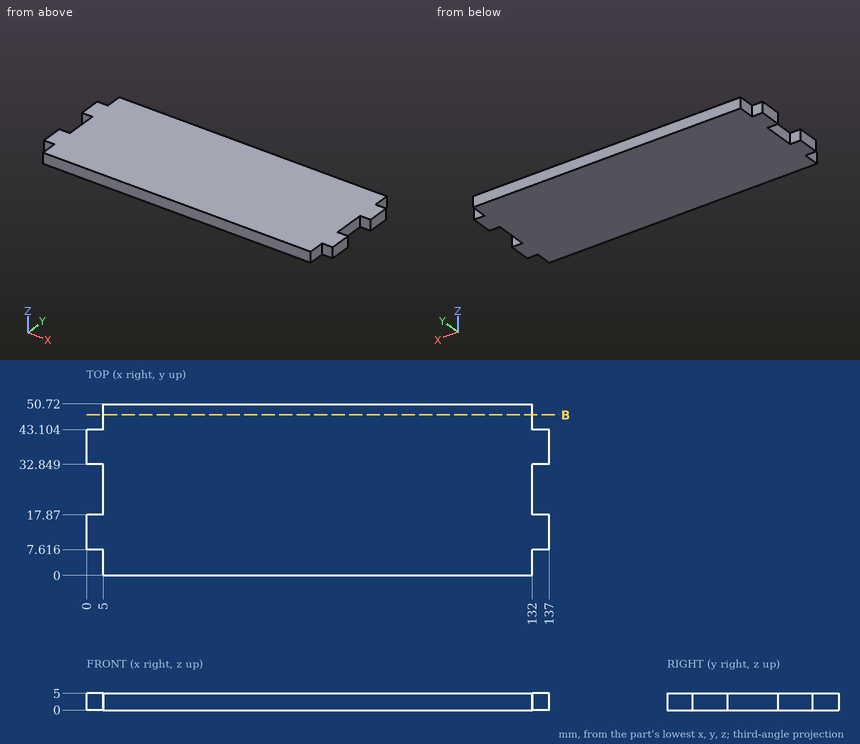
Input: dimensioned drawing with shaded views. Units: mm. Origin: part minimum x, y, z. Round coordinates to 2 decimals unless told otherwise and drop trailing zeros. Order: outer loops, then holes, each group sorted by start corner. A loop starts at its lowest first (then second) coordinate and runs counter-clockwise, first axis right, second up. Notation, with made-up numbers: (-18, -9) -> (12, -9) arc R12 ccw to (12, -4) -> close; hole circle Ø7 at (15, -2). An arc over 180 degrees is marked (long way). Put each result on its own line as item: value. Start each with the question number.
Q1. Line query: probe 1 along X at (y, z) = (19.5, 0.6). Output: solid intervals per line, ascending.
Q2. Section B-B on y = 47.5. Return the cut outline in (x, z), and give its area (3 significant figures).
Q3. First-contact query: pin 1 (2.5 mm diameter, centred on y = 4.5, z = 2, fed in from +X); pin 2 (2.5 mm diameter, centred on x = 134, z = 3, fed in from -Y); pin 3 (2.5 mm diameter, centred on y = 48, z = 2, fed in from -X). Flat tips, straight axial feed; report the tip coordinate or a pass-through.
Ans:
1. probe 1: x = 5 to 132
2. outline: (5, 0) -> (132, 0) -> (132, 5) -> (5, 5) -> close
2. area: 635 mm2
3. pin 1: stops at x = 132
3. pin 2: stops at y = 7.62
3. pin 3: stops at x = 5
